from build123d import *

# Parameters (mm, degrees)
F1_DEPTH = 7


with BuildPart() as f1:
    # F0 (on Top) → F1 (new body)
    with BuildSketch(Plane.XY):
        with BuildLine():
            Line((-7.7118040062, 34.6460978838), (-7.7118040062, -62.2957423329))
            ThreePointArc((-7.7118040062, -62.2957423329), (2.2881959938, -52.2957423329), (12.2881959938, -62.2957423329))
            Line((12.2881959938, -62.2957423329), (12.2881959938, 34.6460978838))
            ThreePointArc((12.2881959938, 34.6460978838), (2.2881959938, 30.8264377713), (-7.7118040062, 34.6460978838))
        make_face()
        with BuildLine():
            ThreePointArc((12.2881959938, -62.2957423329), (2.2881959938, -52.2957423329), (-7.7118040062, -62.2957423329))
            ThreePointArc((-7.7118040062, -62.2957423329), (2.2881959938, -72.2957423329), (12.2881959938, -62.2957423329))
        make_face()
        with BuildLine():
            ThreePointArc((17.2881959938, 45.8264377713), (-3.8355283632, 59.5195017089), (-7.7118040062, 34.6460978838))
            Line((-7.7118040062, 34.6460978838), (-7.7118040062, 41.0087619831))
            ThreePointArc((-7.7118040062, 41.0087619831), (-0.1826338264, 56.647944136), (13.3881959938, 45.8264377713))
            ThreePointArc((13.3881959938, 45.8264377713), (13.1097023584, 43.3556079512), (12.2881959938, 41.0087619831))
            Line((12.2881959938, 41.0087619831), (12.2881959938, 34.6460978838))
            ThreePointArc((12.2881959938, 34.6460978838), (15.9812599314, 39.7027134144), (17.2881959938, 45.8264377713))
        make_face()
        with BuildLine():
            Line((-7.7118040062, 41.0087619831), (-7.7118040062, 34.6460978838))
            ThreePointArc((-7.7118040062, 34.6460978838), (2.2881959938, 30.8264377713), (12.2881959938, 34.6460978838))
            Line((12.2881959938, 34.6460978838), (12.2881959938, 41.0087619831))
            ThreePointArc((12.2881959938, 41.0087619831), (2.2881959938, 34.7264377713), (-7.7118040062, 41.0087619831))
        make_face()
    extrude(amount=F1_DEPTH)


solid = f1.part
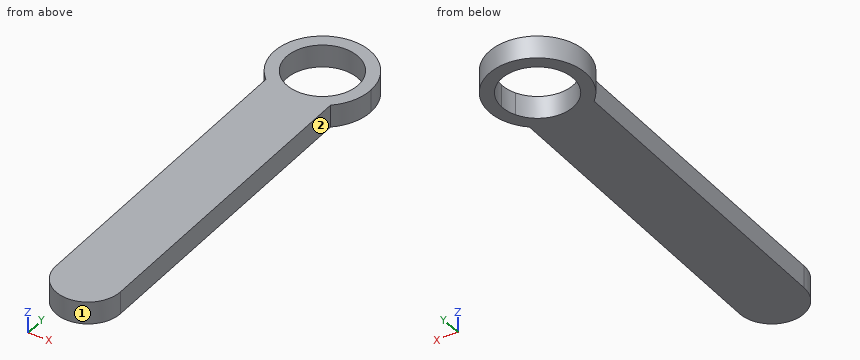
Part model, mm, in its own coordinate system. Face numbers are marked on the shaded views. A direction names the side the tool comes from. Coordinates: 2 decimals unless noted, no trailing zeros. Order: outer loops, then holes, each group sorted by start corner. A loop starts at its lowest first (then second) coordinate and runs counter-clockwise, first axis right, second up. Notation, with made-up numbers: (15.25, 8) - (65.25, 8) arc R17 cw to (65.25, 29) - close; hole circle Ø2 at (-3.75, -29). An arc over 180 degrees is marked (long way). Use CSV: the item, a comma, the result in double quotes.
Item 1: Probe probe 1 along X at (y, z) = (-2, 5.25); probe 2 along X at (y, z) = (47, 3.75); probe 3 along Y at (x, z) = (5.5, 5). List the from-to ranges inside material, lowest first.
Solved:
probe 1,"x = -7.71 to 12.29"
probe 2,"x = -12.67 to -8.75, 13.33 to 17.24"
probe 3,"y = -71.77 to 35.2, 56.45 to 60.48"
Item 2: Saw through at B-B on z = 2.75. Give the cut face in (x, y), and give its area (3 significant figures).
Solved:
outline,"(-7.71, -62.3) arc R10 ccw to (12.29, -62.3) - (12.29, 34.65) arc R15 ccw (long way) to (-7.71, 34.65) - close; hole circle Ø22.2 at (2.29, 45.83)"
area,"2,360 mm²"
Item 3: Saw through at A-A on y = 39. Give the cut face in (x, z), and give its area (3 significant figures).
Solved:
outline,"(-11.07, 0) - (-6.46, 0) - (-6.46, 7) - (-11.07, 7) - close; (11.04, 0) - (15.64, 0) - (15.64, 7) - (11.04, 7) - close"
area,"64.5 mm²"
Item 4: Drop flat-ended pins along their axis: P1, Ø3.5, axis at y = -21, z = 5, coming from the -X side; P2, Ø2, axis at x = 11.5, z = 2.5, coming from the -Y side. Give the stop position or say it passes through.
Solved:
P1,"stops at x = -7.71"
P2,"stops at y = -68"
Item 5: Saw through at D-D on y = -6. Give the cut face in (x, z).
Solved:
outline,"(-7.71, 0) - (12.29, 0) - (12.29, 7) - (-7.71, 7) - close"
Item 6: Saw through at C-C on x = 2.5. Give the cut face in (y, z), and give its area (3 significant figures).
Solved:
outline,"(-72.29, 0) - (34.73, 0) - (34.73, 7) - (-72.29, 7) - close; (56.92, 0) - (60.82, 0) - (60.82, 7) - (56.92, 7) - close"
area,"776 mm²"
Item 7: 3-axis set-ups, long thin cutter, end or side, ignore diameter. For the marked faces 1 and 2: which of +Z, -Z, +X, -X, +Y, -Y reach the whole face in a straight line?
Solved:
face 1,"+Z, -Z, -Y"
face 2,"+Z, -Z, +X, -Y"
